from build123d import *

# Parameters (mm, degrees)
F0_R     = 3.5
F0_R_2   = 3
F1_DEPTH = 3
F2_SIZE  = 0.5
F3_SIZE  = 2


with BuildPart() as f1:
    # F0 (on Front) → F1 (new body)
    with BuildSketch(Plane.XZ):
        with BuildLine():
            ThreePointArc((5, 0), (15, -10), (25, 0))
            ThreePointArc((25, 0), (0, 25), (-25, 0))
            ThreePointArc((-25, 0), (-23.515691, -5.242423), (-19.5034, -8.928571))
            ThreePointArc((-19.5034, -8.928571), (-9.757577, -8.515691), (-5, 0))
            ThreePointArc((-5, 0), (0, 5), (5, 0))
        make_face()
        with Locations((-15, 0)):
            Circle(F0_R, mode=Mode.SUBTRACT)
        with Locations((15, 0)):
            Circle(F0_R, mode=Mode.SUBTRACT)
        with BuildLine():
            ThreePointArc((-5, 0), (-9.757577, -8.515691), (-19.5034, -8.928571))
            ThreePointArc((-19.5034, -8.928571), (-12.820251, -14.739516), (-9.717181, -23.034244))
            Line((-9.717181, -23.034244), (-5.032841, -54.967159))
            ThreePointArc((-5.032841, -54.967159), (-4.20685, -57.729749), (-2, -59.585545))
            Line((-2, -59.585545), (-2, -4.582576))
            ThreePointArc((-2, -4.582576), (-4.1833, -2.738613), (-5, 0))
        make_face()
        with BuildLine():
            ThreePointArc((0, -5), (-1.021548, -4.894532), (-2, -4.582576))
            Line((-2, -4.582576), (-2, -59.585545))
            ThreePointArc((-2, -59.585545), (-1.021246, -59.895297), (0, -60))
            Line((0, -60), (0, -5))
        make_face()
        with Locations((-15, 0)):
            Circle(F0_R)
        with Locations((-15, 0)):
            Circle(F0_R_2, mode=Mode.SUBTRACT)
        with Locations((15, 0)):
            Circle(F0_R)
        with Locations((15, 0)):
            Circle(F0_R_2, mode=Mode.SUBTRACT)
    extrude(amount=F1_DEPTH)

    # F2
    f2_edges = [f1.edges().sort_by_distance(p)[0] for p in [
        (-18, -3, 0),
        (12, -3, 0),
    ]]
    chamfer(f2_edges, length=F2_SIZE)

    # F3
    f3_edges = [f1.edges().sort_by_distance(p)[0] for p in [
        (0, -3, -32.5),
    ]]
    chamfer(f3_edges, length=F3_SIZE)


solid = f1.part
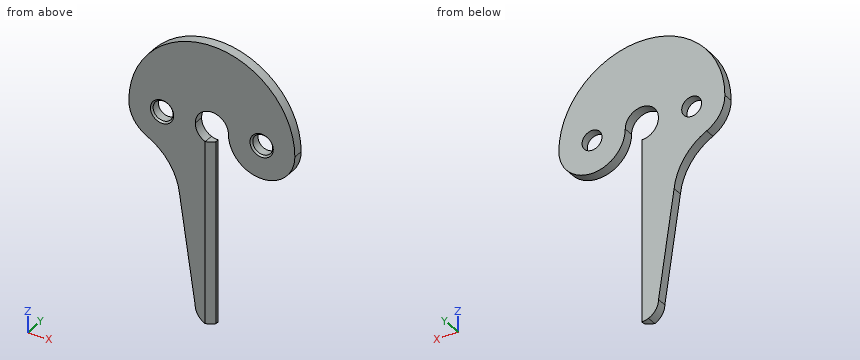
Part model, mm, in its own coordinate system. Coordinates: 2 decimals unless noted, no trailing zeros. Loops run counter-clockwise (first coordinate to the right, second up) from the corner with the lowest first, then second, coordinate; pieces in that order, holes last. Notation, with made-up numbers: (76.25, 23) -> (103.25, 23) arc R18 ccw to (103.25, 29) -> close; hole circle Ø5 at (-37, 66). An arc over 180 degrees is marked (long way). Use a Markdown table: item, result. Add a question column.
Item 1: Band-saw the part on B-B on x = -15. Write the cut outline in (y, z), plus the area to 3 significant figures.
Item 2: Band-saw the part on A-A on x = 15. Write the cut outline in (y, z), plus the area to 4 significant figures.
Item 3: Band-saw the part on C-C on z = -13. Write the cut outline in (x, y).
Item 4: Probe probe 1 along Z at (x, y) = (15, -0.7); probe 2 along Z at (x, y) = (-13, -1); probe 3 along Z at (x, y) = (0, -1.1). List the from-to ranges inside material, lowest first.
Item 5: Band-saw the part on D-D on x = 8. Write the cut outline in (y, z).
Geometry says:
| question | item | result |
|---|---|---|
| 1 | outline | (-3, -12.15) -> (0, -12.15) -> (0, -3) -> (-2.5, -3) -> (-3, -3.5) -> close; (-3, 3.5) -> (-2.5, 3) -> (0, 3) -> (0, 20) -> (-3, 20) -> close |
| 1 | area | 78.2 mm² |
| 2 | outline | (-3, -10) -> (0, -10) -> (0, -3) -> (-2.5, -3) -> (-3, -3.5) -> close; (-3, 3.5) -> (-2.5, 3) -> (0, 3) -> (0, 20) -> (-3, 20) -> close |
| 2 | area | 71.75 mm² |
| 3 | outline | (-14.19, -3) -> (-2, -3) -> (0, -1) -> (0, 0) -> (-14.19, 0) -> close |
| 4 | probe 1 | -10 to -3, 3 to 20 |
| 4 | probe 2 | -14.49 to -2.24, 2.24 to 21.35 |
| 4 | probe 3 | 5 to 25 |
| 5 | outline | (-3, -7.14) -> (0, -7.14) -> (0, 23.69) -> (-3, 23.69) -> close |
